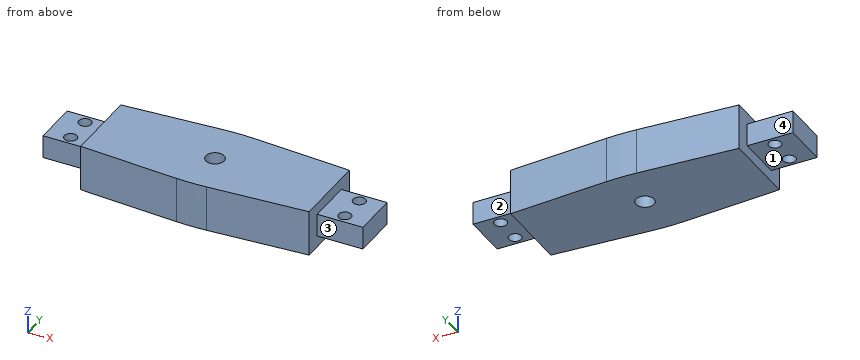
from build123d import *

# Parameters (mm, degrees)
SKETCH1_R           = 4.025
BOSS_EXTRUDE1_DEPTH = 20
FILLET1_R           = 100
SKETCH2_W           = 10
SKETCH2_H           = 20
BOSS_EXTRUDE2_DEPTH = 20
SKETCH3_R           = 2.75
CUT_EXTRUDE1_DEPTH  = 16


with BuildPart() as part:
    # Sketch1 → Boss-Extrude1 (new body)
    with BuildSketch(Plane.XY):
        Polygon((50, 16.695671227), (50, -16.695671227), (0, -20), (-50, -16.695671227), (-50, 16.695671227), (0, 20), align=None)
        Circle(SKETCH1_R, mode=Mode.SUBTRACT)
    extrude(amount=BOSS_EXTRUDE1_DEPTH)

    # Fillet1
    fillet1_edges = [part.edges().sort_by_distance(p)[0] for p in [
        (0, -20, 10),
        (0, 20, 10),
    ]]
    fillet(fillet1_edges, radius=FILLET1_R)

    # Sketch2 → Boss-Extrude2 (add)
    with BuildSketch(Plane(origin=(50, 0, 0), x_dir=(0, 0, -1), z_dir=(1, 0, 0))):
        with Locations((-10, 0)):
            Rectangle(SKETCH2_W, SKETCH2_H)
    boss_extrude2 = extrude(amount=BOSS_EXTRUDE2_DEPTH)

    # Mirror1: Boss-Extrude2 across plane
    add(boss_extrude2.mirror(Plane(origin=(0, 0, 0), x_dir=(0, 0, 1), z_dir=(1, 0, 0))))

    # Sketch3 → Cut-Extrude1 (cut, through all)
    with BuildSketch(Plane(origin=(0, 0, 5), x_dir=(-1, 0, 0), z_dir=(0, 0, -1))):
        with Locations((60, -6)):
            Circle(SKETCH3_R)
        with Locations((60, 6)):
            Circle(SKETCH3_R)
        with Locations((-60, -6)):
            Circle(SKETCH3_R)
        with Locations((-60, 6)):
            Circle(SKETCH3_R)
    extrude(amount=-CUT_EXTRUDE1_DEPTH, mode=Mode.SUBTRACT)


solid = part.part
Can you work these out from the model? Positions are in its coordinate system, mm. Face numbers are marked on the shaded views. A direction names the side the tool comes from. Give positions to 0.01 mm unless a question says otherwise; leave off trailing zeros. Loops run counter-clockwise (first coordinate to the right, second up) from the corner with the lowest first, then second, coordinate; pieces in that order, holes last. Notation, with made-up numbers: (35.25, 47) - (56.25, 47) arc R20 cw to (56.25, 80) - close; hole circle Ø2 at (30, 62). An arc over 180 degrees is marked (long way). Return JSON: item names as keys, results as strings.
1. If I drill on line 1 (Y direction, x = -60, z = 8); line 2 (Y direction, x = 0, z = 10) (3 decimals); line 3 (X direction, y = 7, z = 9), over which ranges is the centre line in solid material (lowest first)?
Output values:
{"line 1": "y = -10 to -8.75, -3.25 to 3.25, 8.75 to 10", "line 2": "y = -19.782 to -4.025, 4.025 to 19.782", "line 3": "x = -70 to -62.56, -57.44 to 57.44, 62.56 to 70"}
2. I want a section at A-A on x = -60. Please give me the cut outline in (y, z).
Output values:
{"outline": "(-10, 5) - (-8.75, 5) - (-8.75, 15) - (-10, 15) - close; (-3.25, 5) - (3.25, 5) - (3.25, 15) - (-3.25, 15) - close; (8.75, 5) - (10, 5) - (10, 15) - (8.75, 15) - close"}
3. I want a section at C-C on y = 6. Please give me the cut outline in (x, z).
Output values:
{"outline": "(-70, 5) - (-62.75, 5) - (-62.75, 15) - (-70, 15) - close; (-57.25, 5) - (-50, 5) - (-50, 0) - (50, 0) - (50, 5) - (57.25, 5) - (57.25, 15) - (50, 15) - (50, 20) - (-50, 20) - (-50, 15) - (-57.25, 15) - close; (62.75, 5) - (70, 5) - (70, 15) - (62.75, 15) - close"}
4. I want a section at B-B on y = 0. Please give me the cut outline in (x, z) (3 decimals), and give its area (3 significant figures).
Output values:
{"outline": "(-70, 5) - (-50, 5) - (-50, 0) - (-4.025, 0) - (-4.025, 20) - (-50, 20) - (-50, 15) - (-70, 15) - close; (4.025, 0) - (50, 0) - (50, 5) - (70, 5) - (70, 15) - (50, 15) - (50, 20) - (4.025, 20) - close", "area": "2,240 mm²"}
5. For the marked faces 1, 2, 3 and 4, which set-ups out of +Z, -Z, +X, -X, +Y, -Y let a thin tool reach every point of the face, with its end or its side?
Output values:
{"face 1": "-Z, -X, +Y, -Y", "face 2": "+Z, -Z, +X, +Y", "face 3": "+Z, -Z, +X, -Y", "face 4": "+Z, -Z, -X, +Y"}
6. I'm going to push flat-ended pins straight in: pin 1 Ø3 at (x, z) = (-63, 11) entering from +Y; pin 2 Ø3 at (x, z) = (-63, 9) entering from -Y; pin 3 Ø1.5 at (x, z) = (47, 3) entering from +Y. Where does each tip first touch, or does it pass through?
Output values:
{"pin 1": "stops at y = 10", "pin 2": "stops at y = -10", "pin 3": "stops at y = 16.94"}
7. I want a section at D-D on z = 8. Please give me the cut outline in (x, y) (3 decimals).
Output values:
{"outline": "(-70, -10) - (-50, -10) - (-50, -16.696) - (-6.594, -19.564) arc R100 ccw to (6.594, -19.564) - (50, -16.696) - (50, -10) - (70, -10) - (70, 10) - (50, 10) - (50, 16.696) - (6.594, 19.564) arc R100 ccw to (-6.594, 19.564) - (-50, 16.696) - (-50, 10) - (-70, 10) - close; hole circle Ø5.5 at (-60, -6); hole circle Ø5.5 at (-60, 6); hole circle Ø8.05 at (0, 0); hole circle Ø5.5 at (60, -6); hole circle Ø5.5 at (60, 6)"}
